Autodesk Inventor part; units mm, degrees
ref_plane "Work Plane1" through (34.2931, 25.9114, -33.2342) normal (0, 1, 0) x (-1, 0, 0)
ref_plane "작업 평면2" through (4.5431, 25.6014, -33.2342) normal (0, 0, 1) x (1, 0, 0)
ref_plane "YZ Plane" through (0, 0, 0) normal (1, 0, 0) x (0, 1, 0)
ref_plane "Work Plane1" through (34.2931, 25.9114, -33.2342) normal (0, 1, 0) x (-1, 0, 0)
sketch "Sketch2" plane through (34.2931, 25.9114, -33.2342) normal (0, 1, 0) x (-1, 0, 0)
  circle A0 centre (9.75, 7.1) radius 0.7835
  circle A1 centre (16.85, 0) radius 0.7835
  circle A2 centre (9.75, -7.1) radius 0.7835
  circle A3 centre (2.65, 0) radius 0.7835
  circle A4 centre (4.7295, -5.0205) radius 0.7835
  circle A5 centre (14.7705, -5.0205) radius 0.7835
  circle A6 centre (14.7705, 5.0205) radius 0.7835
  circle A7 centre (4.7295, 5.0205) radius 0.7835
  circle A8 centre (9.75, 0) radius 3.8
  circle A9 centre (9.75, 0) radius 9.75
  circle A10 centre (9.75, 0) radius 2.75
  line L0 (29.75, -10.5) -> (29.75, 10.5)
  line L1 (29.75, -10.5) -> (24.75, -10.5)
  line L2 (29.75, 10.5) -> (24.75, 10.5)
  line L3 (24.75, -10.5) -> (9.2707, -9.7382)
  line L4 (24.75, 10.5) -> (9.2707, 9.7382)
  circle A11 centre (9.75, -7.1) radius 1.05
  circle A12 centre (16.85, 0) radius 1.05
  circle A13 centre (9.75, 7.1) radius 1.05
  circle A14 centre (2.65, 0) radius 1.05
  point P0 (34.2931, 33.2342)
  point P1 (29.75, 0)
  dimension "d2" = 5.5
  dimension "d4" = 21
  dimension "d5" = 5
  dimension "d6" = 20
  dimension "d36" = 2.1
extrude "Plate2" add sketch "Sketch2" along normal blind 1.5 contours A4 | A5 | A6 | A7 | A8 | A9 | A9 L4 L2 L0 L1 L3
sketch "Sketch3" plane through (6.0431, 27.4114, -43.7342) normal (-1, 0, 0) x (0, -1, 0)
  line L0 (0, 21) -> (0, 0)
  line L1 (0, 0) -> (55, 0)
  line L2 (55, 0) -> (55, 21)
  line L3 (55, 21) -> (0, 21)
edge flange "Flange1" height 55 angle 90 thickness 1.5 bend radius 0.31 thickness toward (-1, 0, 0) relief tear relief width 1.5 relief depth 0.75 edges at (4.5431, 25.9114, -33.2342) wall of the first edge with corners at (6.0431, 27.4114, -22.7342) (6.0431, 27.4114, -43.7342) (6.0431, -27.5886, -43.7342) (6.0431, -27.5886, -22.7342)
bend "Bend1"
corner "Corner1"
sketch "Sketch4" plane through (4.5431, -26.0886, -43.7342) normal (0, -1, 0) x (1, 0, 0)
  line L0 (0, 21) -> (0, 0)
  line L1 (0, 0) -> (30, 0)
  line L2 (30, 0) -> (30, 21)
  line L3 (30, 21) -> (0, 21)
edge flange "Flange2" height 30 angle 90 thickness 1.5 bend radius 0.31 thickness toward (0, -1, 0) relief tear relief width 1.5 relief depth 0.75 edges at (6.0431, -27.5886, -33.2342) wall of the first edge with corners at (4.5431, -26.0886, -22.7342) (4.5431, -26.0886, -43.7342) (34.5431, -26.0886, -43.7342) (34.5431, -26.0886, -22.7342)
bend "Bend2"
corner "Corner2"
sketch "Sketch5" plane through (34.5431, -27.5886, -43.7342) normal (0, -1, 0) x (1, 0, 0)
  circle A0 centre (-10, 10.5) radius 3.8
  circle A1 centre (-10, 10.5) radius 3.85
  point P0 (-34.5431, 43.7342)
  dimension "d37" = 7.7
extrude "Cut1" cut sketch "Sketch5" against normal blind 1.5 contours A0 | A1
sketch "Sketch6" plane through (34.5431, -27.5886, -43.7342) normal (0, -1, 0) x (1, 0, 0)
  circle A0 centre (-10, 17.525) radius 0.7835
  circle A1 centre (-2.975, 10.5) radius 0.7835
  circle A2 centre (-10, 3.475) radius 0.7835
  circle A3 centre (-17.025, 10.5) radius 0.7835
  circle A4 centre (-10, 10.5) radius 9.75
  line L0 (-25, 21) -> (-9.5207, 20.2382)
  line L1 (-9.5207, 0.7618) -> (-25, 0)
  line L2 (-28.19, 21) -> (0, 21)
  line L3 (0, 21) -> (0, 0)
  line L4 (0, 0) -> (-28.19, 0)
  line L5 (-28.19, 21) -> (-30, 21)
  line L6 (-30, 0) -> (-28.19, 0)
  circle A5 centre (-2.975, 10.5) radius 1.05
  circle A6 centre (-10, 17.525) radius 1.05
  circle A7 centre (-17.025, 10.5) radius 1.05
  circle A8 centre (-10, 3.475) radius 1.05
  point P0 (-34.5431, 43.7342)
  dimension "d35" = 2.1
extrude "Cut2" cut sketch "Sketch6" against normal blind 1.5 contours A0 | A1 | A2 | A3 | A4 L0 L2 L3 L4 L1 | A5 | A6 | A7 | A8
ref_plane "작업 평면2" through (4.5431, 25.6014, -33.2342) normal (0, 0, 1) x (1, 0, 0)
sketch "Sketch7" plane through (6.0431, 25.6014, -22.7342) normal (1, 0, 0) x (0, 0, -1)
  circle A0 centre (5.5, -13.69) radius 0.7835
  circle A1 centre (15.5, -13.69) radius 0.7835
  circle A2 centre (5.5, -39.19) radius 0.7835
  circle A3 centre (15.5, -39.19) radius 0.7835
  circle A4 centre (5.5, -13.69) radius 1.05
  circle A5 centre (15.5, -13.69) radius 1.05
  circle A6 centre (5.5, -39.19) radius 1.05
  circle A7 centre (15.5, -39.19) radius 1.05
  point P0 (-22.7342, -25.6014)
  dimension "d34" = 2.1
extrude "Cut3" cut sketch "Sketch7" against normal blind 1.5 contours A0 | A1 | A2 | A3 | A4 | A5 | A6 | A7
equation "\"d28\" = Thickness"
equation "\"d30\" = Thickness"
equation "\"d32\" = Thickness"
equation "\"d7\" = Thickness"
equation "\"d8\" = BendReliefWidth"
equation "\"d9\" = BendReliefDepth"
equation "\"d10\" = MinimumRemnant"
equation "\"d11\" = TransitionRadius"
equation "\"d14\" = BendRadius"
equation "\"d15\" = CornerReliefSize"
equation "\"d16\" = GapSize"
equation "\"d17\" = JacobiRadiusSize"
equation "\"d18\" = BendReliefWidth"
equation "\"d19\" = BendReliefDepth"
equation "\"d20\" = MinimumRemnant"
equation "\"d21\" = TransitionRadius"
equation "\"d24\" = BendRadius"
equation "\"d25\" = CornerReliefSize"
equation "\"d26\" = GapSize"
equation "\"d27\" = JacobiRadiusSize"
equation "\"BendReliefWidth\" = Thickness"
equation "\"BendReliefDepth\" = 0.5 * Thickness"
equation "\"CornerReliefSize\" = 4 * Thickness"
equation "\"MinimumRemnant\" = 2 * Thickness"
equation "\"TransitionRadius\" = BendRadius"
equation "\"JacobiRadiusSize\" = BendRadius"
equation "\"GapSize\" = Thickness"
properties part number "ㄷ_frame_2" material "Aluminum 6061"
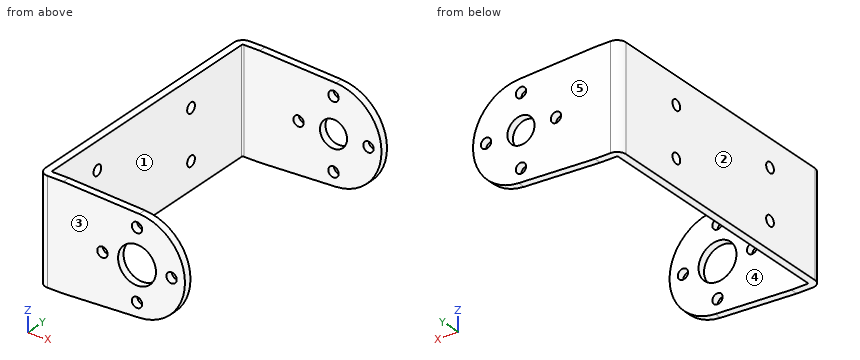
The listing builds one solid part. Answer for the finished solid, in the listing's coordinates (mm). Face numbers are marked on the shaded views. A direction names the side the tool comes from. Give positions to 0.01 mm unless a question says otherwise; leave off trailing zeros. Write each loop counter-clockwise with the first axis right and the second up, starting at its lowest first coordinate (ties: lowest second). Pieces come first, ordered by that corner, then holes.
Item 1: Find the intervals of material crossed by line 1 along Y through (x, z) = (11.75, -34.5); line 2 along X through (y, z) = (16, -34.25); line 3 along Y through (x, z) = (22.75, -35.75), in increasing order.
Item 2: Section C-C, the plane y = 18 is taken. Write down the section's boundary in (x, z), plus the area to 3 significant figures.
Item 3: Section A-A, the plane x = 8.5 is taken. Write down the section's boundary in (y, z), plus the area to 3 significant figures.
Item 4: Which of the six approach directions +Z, -Z, +X, -X, +Y, -Y give full straight-line access (tool end or side, diameter ignored) to the marked faces 4 and 5?
Item 5: Section D-D, the plane x = 26.75 is taken. Write down the section's boundary in (y, z).
Item 6: Section B-B, the plane x = 31.25 is taken. Write down the section's boundary in (y, z).
Item 7: Determine the mould class of the marked faces 1, 2 and 3 for opening direction Y: released by +Y, released by -Y, zero draft, split by the parting line, or undercut.
Item 8: Flat-ended cylindrical pins translate along their axes: P1, Ø1.9, axis at y = -13.59, z = -28.23, coming from the +X side; P2, Ø2.5, axis at y = -13.59, z = -38.23, coming from the +X side. Find the tip coordinate at first contact, or state that the pin passes through.
Completed:
1. line 1: y = -27.59 to -26.09, 25.91 to 27.41
1. line 2: x = 4.54 to 6.04
1. line 3: y = 25.91 to 27.41
2. outline: (4.54, -43.73) - (6.04, -43.73) - (6.04, -22.73) - (4.54, -22.73) - close
2. area: 31.5 mm2
3. outline: (-27.59, -43.73) - (-26.09, -43.73) - (-26.09, -22.73) - (-27.59, -22.73) - close; (25.91, -43.73) - (27.41, -43.73) - (27.41, -22.73) - (25.91, -22.73) - close
3. area: 63.0 mm2
4. face 4: +Z, -Z, +X
4. face 5: +Z, -Z, +X, -X, +Y
5. outline: (-27.59, -42.73) - (-26.09, -42.73) - (-26.09, -36.39) - (-27.59, -36.39) - close; (-27.59, -30.08) - (-26.09, -30.08) - (-26.09, -23.74) - (-27.59, -23.74) - close; (25.91, -42.73) - (27.41, -42.73) - (27.41, -34.87) - (25.91, -34.87) - close; (25.91, -31.59) - (27.41, -31.59) - (27.41, -23.74) - (25.91, -23.74) - close
6. outline: (-27.59, -40.31) - (-26.09, -40.31) - (-26.09, -34.23) - (-27.59, -34.23) - close; (-27.59, -32.23) - (-26.09, -32.23) - (-26.09, -26.16) - (-27.59, -26.16) - close; (25.91, -40.31) - (27.41, -40.31) - (27.41, -34.21) - (25.91, -34.21) - close; (25.91, -32.26) - (27.41, -32.26) - (27.41, -26.16) - (25.91, -26.16) - close
7. face 1: undercut
7. face 2: zero draft
7. face 3: released by -Y
8. P1: passes through
8. P2: stops at x = 6.04
